The model under review builds one solid part; all positions refer to its coordinate system, in mm. A direction names the side the tool comes from. Round coordinates to 2 decimals unless told otherwise and drop trailing zeros. Order: outer loops, then holes, each group sorted by start corner. A loop starts at its lowest first (then second) coordinate and runs counter-clockwise, first axis right, second up. Notation, with made-up numbers: (-5.75, 52) -> (2.25, 52) arc R22 cw to (2.25, 86) -> close; hole circle Ø10 at (-21, 61.25). An arc over 180 degrees is marked (long way). Use a Markdown table: item, result. Add a question column.
Autodesk Inventor part; units mm, degrees
ref_plane "Work Plane1" through (-9, 10, 0) normal (1, 0, 0) x (0, 1, 0)
ref_plane "XZ Plane" through (0, 0, 0) normal (0, 1, 0) x (-1, 0, 0)
ref_plane "XY Plane" through (0, 0, 0) normal (0, 0, 1) x (1, 0, 0)
sketch "Sketch1" plane through (0, 0, 0) normal (0, 0, 1) x (1, 0, 0)
  line L0 (0, 60) -> (0, -60)
  line L1 (0, -60) -> (15, -60)
  line L2 (9, 60) -> (0, 60)
  line L3 (9, -40) -> (15, -40)
  line L4 (9, -40) -> (9, 60)
  line L5 (15, -40) -> (15, -60)
  point P0 (0, 0)
  point P1 (0, 0)
  dimension "d17" = 18
  dimension "d18" = 20
  dimension "d19" = 30
  dimension "d42" = 100
revolve "Revolution1" add sketch "Sketch1" angle 360 about axis through (0, 60, 0) along (0, -1, 0)
sketch "Sketch4" plane through (0, 60, 0) normal (0, 1, 0) x (1, 0, 0)
  point P0 (0, 0)
  point P1 (0, 0)
hole "Hole1" at (0, 60, 0) direction (0, -1, 0) diameter 6.647 depth 22.2 tip angle 118
chamfer "Chamfer1" distance 1 angle 45 1 edges at (-9, 60, 0)
ref_plane "Work Plane1" through (-9, 10, 0) normal (1, 0, 0) x (0, 1, 0)
sketch "Sketch5" plane through (-9, 10, 0) normal (1, 0, 0) x (0, 1, 0)
  line L0 (-50, 9) -> (-50, -9)
  line L1 (49, -9) -> (49, 9)
  line L2 (35, 0) -> (15, 0) construction
  line L3 (35, -3) -> (15, -3)
  line L4 (15, 3) -> (35, 3)
  arc A0 (35, -3) -> (35, 3) centre (35, 0) ccw
  arc A1 (15, 3) -> (15, -3) centre (15, 0) ccw
  line L5 (50, 8) -> (50, -8)
  point P0 (-10, 0)
  point P1 (25, 0)
  dimension "d36" = 6
  dimension "d37" = 20
  dimension "d39" = 15
extrude "Extrusion3" cut sketch "Sketch5" along normal blind 3
properties part number "приводной вал"
Q1. Add section A-A (y = 41). Write out the cut boundary in (x, z).
Q2. Add section B-B (y = 14). Write out the cut boundary in (x, z), then the cut area to 3 significant figures.
Q3. Mouldability with a two-part tool opening along Z and no side actions: class faces 1 (the cylindrical face through (1.27, 48.74, 3.07)), 2 (the cylindrical face through (8.584, 10.193, -2.703)), 3 (the flat face through (6.5, -40, -6.5)) as pulls with the +Z half, pulls with the -Z half, needs draft (parallel to the pull), parting line crosses it, or undercut.
Q4. Wall thickness on line 1 (Z direction, x = -0.25, y = 50.5); line 2 (X direction, y = 51.25, z = 0); line 3 (Y direction, x = -0.25, z = 10): over which ranges is each line inside the solid? List them lowest first. Write a range as [from, to].
Q5. Machinability: for faces 4 (the flat face through (-6, 35, 0)), 5 (the flat face through (0, -60, 0)), which of the approach directions +Z, -Z, +X, -X, +Y, -Y give a long, thin tool a straight path to every point of the face, cutting with its end or side? Answer none if there is none.
Q6. Insertion check: pin 1 (1.2 mm diameter, centred on x = -7.5, y = 30, fed in from +Z); pin 2 (5.5 mm diameter, centred on x = 0, z = 0, fed in from +Y); pin 3 (3 mm diameter, centred on x = 1.5, z = 0.5, fed in from +Y). Each pin has a flat end and moves straight along its axis. Give the tip position at first contact, or say it passes through.
Report:
| question | item | result |
|---|---|---|
| 1 | outline | (-8.49, -3) arc R9 ccw (long way) to (-8.49, 3) -> (-6, 3) -> (-6, -3) -> close; hole circle Ø6.65 at (0, 0) |
| 2 | outline | circle Ø18 at (0, 0) |
| 2 | area | 254 mm² |
| 3 | face 1 | undercut |
| 3 | face 2 | parting line crosses it |
| 3 | face 3 | needs draft |
| 4 | line 1 | z = [-9, -3.31], [3.31, 9] |
| 4 | line 2 | x = [-9, -3.32], [3.32, 9] |
| 4 | line 3 | y = [-60, -40] |
| 5 | face 4 | -X |
| 5 | face 5 | +Z, -Z, +X, -X, -Y |
| 6 | pin 1 | stops at z = 5.78 |
| 6 | pin 2 | stops at y = 37.46 |
| 6 | pin 3 | stops at y = 37.65 |
